Build history of the part. All positions in model axes, mm. A direction names the side the tool comes from. Round coordinates to 2 decimals unless told otherwise and drop trailing zeros. Write each loop counter-clockwise with the first axis right and the second up, starting at its lowest first coordinate (ties: lowest second). Pieces come first, ordered by that corner, then holes. Notation, with made-up numbers: M 86,-38 L 120,-38 A5 cw 120,-34 Z; hole C 21,-36.75 d5. An arc over 180 degrees is marked long. Write item = value, one per line.
from build123d import *

# Parameters (mm, degrees)
SKETCH1_W           = 74.93
SKETCH1_H           = 39.878
BOSS_EXTRUDE1_DEPTH = 18.034
SKETCH2_R           = 1.5
CUT_EXTRUDE1_DEPTH  = 18.034
SKETCH3_W           = 65
SKETCH3_H           = 18
CUT_EXTRUDE2_DEPTH  = 17


with BuildPart() as part:
    # Sketch1 → Boss-Extrude1 (new body)
    with BuildSketch(Plane.XY):
        Rectangle(SKETCH1_W, SKETCH1_H)
    extrude(amount=BOSS_EXTRUDE1_DEPTH)

    # Sketch2 → Cut-Extrude1 (cut)
    with BuildSketch(Plane.XY.offset(18.034)):
        with Locations((0, -9.9695)):
            Circle(SKETCH2_R)
        with Locations((0, 9.9695)):
            Circle(SKETCH2_R)
    extrude(amount=-CUT_EXTRUDE1_DEPTH, mode=Mode.SUBTRACT)

    # Sketch3 → Cut-Extrude2 (cut)
    with BuildSketch(Plane.XY.offset(18.034)):
        with Locations((0, 9.9695)):
            Rectangle(SKETCH3_W, SKETCH3_H)
        with Locations((0, -9.9695)):
            Rectangle(SKETCH3_W, SKETCH3_H)
    extrude(amount=-CUT_EXTRUDE2_DEPTH, mode=Mode.SUBTRACT)


solid = part.part
1. Band-saw the part on D-D (x = -23). List the corners of the cut face in (y, z), plus the area to 3 significant figures.
Responses:
outline = M -19.94,0 L 19.94,0 L 19.94,18.03 L 18.97,18.03 L 18.97,1.03 L 0.97,1.03 L 0.97,18.03 L -0.97,18.03 L -0.97,1.03 L -18.97,1.03 L -18.97,18.03 L -19.94,18.03 Z
area = 107 mm²
2. Tool access for faces 1 (the face through (0, 18.97, 10)), 2 (the face through (-0.195, 11.457, 0.524)): list every direction of +Z, -Z, +X, -X, +Y, -Y with a clear straight run to the whole face (end or side of a thin tool).
Responses:
face_1 = +Z
face_2 = +Z, -Z
3. Band-saw the part on C-C (y = 5). List the corners of the cut face in (x, z) (3 decimals).
Responses:
outline = M -37.465,0 L 37.465,0 L 37.465,18.034 L 32.5,18.034 L 32.5,1.034 L -32.5,1.034 L -32.5,18.034 L -37.465,18.034 Z
4. Band-saw the part on A-A (x = 0). List the corners of the cut face in (y, z).
Responses:
outline = M -19.94,0 L -11.47,0 L -11.47,1.03 L -18.97,1.03 L -18.97,18.03 L -19.94,18.03 Z; M -8.47,0 L 8.47,0 L 8.47,1.03 L 0.97,1.03 L 0.97,18.03 L -0.97,18.03 L -0.97,1.03 L -8.47,1.03 Z; M 11.47,0 L 19.94,0 L 19.94,18.03 L 18.97,18.03 L 18.97,1.03 L 11.47,1.03 Z
5. Mould opens along Y. For faces 3 (the face through (0, 0.97, 10)), 4 (the face through (-1, -19.939, 9)), 5 (the face through (-1, 19.939, 9)) say: pulls with the +Y half, pulls with the -Y half, needs draft (parallel to the pull), parting line crosses it, or undercut.
Responses:
face_3 = undercut
face_4 = pulls with the -Y half
face_5 = pulls with the +Y half
6. Probe probe 1 along Y at (x, z) = (-2.5, 3); probe 2 along Y at (x, z) = (0, 0.45); probe 3 along X at (y, z) = (4.5, 2.5) (3 decimals). List the from-to ranges inside material, lowest first.
Responses:
probe_1 = -19.94 to -18.97, -0.97 to 0.97, 18.97 to 19.94
probe_2 = -19.94 to -11.47, -8.47 to 8.47, 11.47 to 19.94
probe_3 = -37.465 to -32.5, 32.5 to 37.465
7. Flat gauge pin, fed straight in: pin 1 (2.5 mm diameter, centred on x = 0, y = -9.97, fed in from -Z). Where does the tip first touch, or does it go through?
Responses:
pin_1 = through
8. Band-saw the part on B-B (z = 7.75). List the corners of the cut face in (x, y) (1 decimal), plus the area to 3 significant figures.
Responses:
outline = M -37.5,-19.9 L 37.5,-19.9 L 37.5,19.9 L -37.5,19.9 Z; hole M -32.5,-19 L 32.5,-19 L 32.5,-1 L -32.5,-1 Z; hole M -32.5,1 L 32.5,1 L 32.5,19 L -32.5,19 Z
area = 648 mm²
